```python
from build123d import *

# Parameters (mm, degrees)
SKETCH1_W           = 381
SKETCH1_H           = 2743.2
BOSS_EXTRUDE1_DEPTH = 50.8
SKETCH2_R           = 63.5
SKETCH2_R_2         = 50.8
BOSS_EXTRUDE2_DEPTH = 50.8
FILLET1_R           = 25.4


with BuildPart() as part:
    # Sketch1 → Boss-Extrude1 (new body)
    with BuildSketch(Plane(origin=(0, 0, 0), x_dir=(1, 0, 0), z_dir=(0, 1, 0))):
        Rectangle(SKETCH1_W, SKETCH1_H)
    extrude(amount=BOSS_EXTRUDE1_DEPTH)

    # Sketch2 → Boss-Extrude2 (add)
    # profile 1 of 3: a face of its own
    with BuildSketch(Plane.XY.offset(1371.6)):
        with BuildLine():
            ThreePointArc((92.766835976, 530.71784895), (78.777173297, 542.88645519), (68.898941042, 558.577413324))
            Line((68.898941042, 558.577413324), (-190.5, 50.8))
            Line((-190.5, 50.8), (-152.4, 50.8))
            Line((-152.4, 50.8), (92.766835976, 530.71784895))
        make_face()
    # profile 2 of 3: a face of its own
    with BuildSketch(Plane.XY.offset(1371.6)):
        with BuildLine():
            Line((152.4, 50.8), (190.5, 50.8))
            Line((190.5, 50.8), (190.5, 584.2))
            ThreePointArc((190.5, 584.2), (180.127911685, 549.419617598), (152.4, 526.001288674))
            Line((152.4, 526.001288674), (152.4, 50.8))
        make_face()
    # profile 3 of 3: a face of its own
    with BuildSketch(Plane.XY.offset(1371.6)):
        with Locations((127, 584.2)):
            Circle(SKETCH2_R)
        with Locations((127, 584.2)):
            Circle(SKETCH2_R_2, mode=Mode.SUBTRACT)
    boss_extrude2 = extrude(amount=-BOSS_EXTRUDE2_DEPTH)

    # Mirror1: Boss-Extrude2 across plane
    add(boss_extrude2.mirror(Plane.XY))

    # Fillet1
    fillet1_edges = [part.edges().sort_by_distance(p)[0] for p in [
        (-152.4, 50.8, 1346.2),
        (152.4, 50.8, 1346.2),
        (-152.4, 50.8, -1346.2),
        (152.4, 50.8, -1346.2),
    ]]
    fillet(fillet1_edges, radius=FILLET1_R)


solid = part.part
```
Design review of the part built by this model. Coordinates are the model's own, in mm. A direction names the side the tool comes from. Coordinates: 2 decimals unless noted, no trailing zeros. Order: outer loops, then holes, each group sorted by start corner. A loop starts at its lowest first (then second) coordinate and runs counter-clockwise, first axis right, second up. Notation, with made-up numbers: (36, -31) - (84, -31) arc R23 cw to (84, -1) - close; hole circle Ø3 at (-38, 84.5). An arc over 180 degrees is marked (long way). One line per question, with ' | ' between items.
Q1. Consider section A-A, the plane y = 355. Give the boundary of the cut face in (x, z), then the cut area to 3 significant figures.
Answer key:
outline: (-35.1, -1371.6) - (3, -1371.6) - (3, -1320.8) - (-35.1, -1320.8) - close; (-35.1, 1320.8) - (3, 1320.8) - (3, 1371.6) - (-35.1, 1371.6) - close; (152.4, -1371.6) - (190.5, -1371.6) - (190.5, -1320.8) - (152.4, -1320.8) - close; (152.4, 1320.8) - (190.5, 1320.8) - (190.5, 1371.6) - (152.4, 1371.6) - close | area: 7,740 mm2
Q2. The part is to be moulded in two halves that separate along Z. For faces 1 (the flat face through (-43, 277, -1371.6)), 2 (the flat face through (-43, 277, 1371.6)), 3 (the flat face through (-1, 351, -1320.8)), 4 (the flat face through (-1, 351, 1320.8)), say which applies: +Z half, -Z half, draft (parallel to the pull), parting line (faces both ways), or undercut.
Answer key:
face 1: -Z half | face 2: +Z half | face 3: undercut | face 4: undercut
Q3. To check wall thickness, follow line 1 along X through (y, z) = (584, -1342); line 2 along Z through (x, y) = (153, 206); line 3 along Y through (x, z) = (157, -301.5). State the ranges of each line that lie inside material, in increasing order.
Answer key:
line 1: x = 63.5 to 76.2, 177.8 to 190.5 | line 2: z = -1371.6 to -1320.8, 1320.8 to 1371.6 | line 3: y = 0 to 50.8
Q4. For faces 5 (the flat face through (190.5, 31, -413)), 6 (the flat face through (-21.96, 306.14, -1346.56)), list the 3-axis set-ups (+Z, -Z, +X, -X, +Y, -Y) from which the entire face can be reached by the end or side of a thin tool; tool diameter is ignored.
Answer key:
face 5: +Z, -Z, +X, +Y, -Y | face 6: +Z, -Z
Q5. Clearance check with flat-ended pins moving along their axes: pin 1 Ø12 at (x, z) = (9, 105.5) entering from +Y; pin 2 Ø12 at (x, z) = (-63, -256) entering from -Y. State where each tip first meets the part, or that it passes through.
Answer key:
pin 1: stops at y = 50.8 | pin 2: stops at y = 0
Q6. Consider section C-C, the plane z = 512. Give the boundary of the cut face in (x, y).
Answer key:
outline: (-190.5, 0) - (190.5, 0) - (190.5, 50.8) - (-190.5, 50.8) - close
Q7. Consider section B-B, the plane x = -65. Give the boundary of the cut face in (y, z).
Answer key:
outline: (0, -1371.6) - (50.8, -1371.6) - (50.8, 1371.6) - (0, 1371.6) - close; (221.89, -1371.6) - (296.47, -1371.6) - (296.47, -1320.8) - (221.89, -1320.8) - close; (221.89, 1320.8) - (296.47, 1320.8) - (296.47, 1371.6) - (221.89, 1371.6) - close
